The listing builds one solid part. Answer for the finished solid, in the listing's coordinates (mm). A direction names the side the tool comes from. Give positions to 0.01 mm unless a question says otherwise; leave off trailing zeros. Loops run counter-clockwise (first coordinate to the right, second up) from the corner with the lowest first, then second, coordinate; pieces in that order, holes last.
Item 1: Consider line 1 along X through (y, z) = (-26, 5.25); line 2 along Y through (x, z) = (21.5, 3.75); line 3 along Z through (x, y) = (40, -47). Determine where each line is inside the solid, lowest interval first.
Item 2: Section D-D, the plane x = 31.5 is taken. Give the vertices of the cut face in (y, z), and give its area (3 significant figures).
Item 3: Each of these flat-tipped pins is pushed along its axis until it touches: pin 1 Ø5.5 at (x, z) = (35.5, 9) entering from -Y; pin 2 Ø3 at (y, z) = (-17, 20) entering from +X; pin 3 Ø3 at (y, z) = (-47, 20) entering from -X; pin 4 Ø1.1 at (x, y) = (38.5, -44.5) entering from +Z. Where does it stop, or does it pass through?
Item 4: Section C-C, the plane y = 12.4 is taken. Give the vertices of the cut face in (x, z).
Item 5: The mould has two halves that part along Z. Classify faces 1 (the face through (-41.1, -16.6, 0.8)), 2 (the face through (-36.859, -45.014, 3.193)), 3 (the face through (-31.155, 16.362, 19.521)): pulls with the +Z half, pulls with the -Z half, needs draft (parallel to the pull), parting line crosses it, or undercut.
Item 6: A tool of negligible diameter and unlimited length cuts with its end or side. For faces 4 (the face through (-35, 12, 14.6)), 5 (the face through (-36, -9, 11)), 6 (the face through (-38.4, -46, 7.9)), 7 (the face through (30, 17, 19.6)), 8 (the face through (42, -17, 13)), from which of +Z, -Z, +X, -X, +Y, -Y can it reach the whole face along a straight path? Write none if from no direction.
Item 7: Section B-B, the plane x = 13 is taken. Give the vertices of the cut face in (y, z), and give its area (3 significant figures).
Item 8: Section A-A, the plane y = -47 is taken. Give the vertices of the cut face in (x, z), and give its area (3 significant figures).
from build123d import *

# Parameters (mm, degrees)
PAD011_DEPTH    = 23
POCKET004_DEPTH = 5
SKETCH018_R     = 1.25
POCKET005_DEPTH = 84.001
SKETCH019_R     = 1.25
POCKET006_DEPTH = 5
CHAMFER_SIZE    = 1.3
PAD015_DEPTH    = 2
FILLET004_R     = 2.9
FILLET005_R     = 1.9
SKETCH023_W     = 6
SKETCH023_H     = 10
SKETCH023_W_2   = 7
PAD016_DEPTH    = 9
CHAMFER001_SIZE = 8.7
SKETCH024_R     = 1.15
POCKET007_DEPTH = 7


with BuildPart() as part:
    # Sketch015 → Pad011 (new body)
    with BuildSketch(Plane.XY):
        with BuildLine():
            ThreePointArc((-39, 18.5), (-41.12132, 17.62132), (-42, 15.5))
            Line((-42, -51.5), (-42, 15.5))
            Line((-39, -51.5), (-42, -51.5))
            Line((-39, 15.5), (-39, -51.5))
            Line((-39, 15.5), (39, 15.5))
            Line((39, -51.5), (39, 15.5))
            Line((42, -51.5), (39, -51.5))
            Line((42, 15.5), (42, -51.5))
            ThreePointArc((42, 15.5), (41.12132, 17.62132), (39, 18.5))
            Line((-39, 18.5), (39, 18.5))
        make_face()
    extrude(amount=PAD011_DEPTH)

    # Sketch017 (on Face10 of Pad011) → Pocket004 (cut)
    with BuildSketch(Plane(origin=(0, 18.5, 0), x_dir=(-1, 0, 0), z_dir=(0, 1, 0))):
        with BuildLine():
            Line((-25.5, 23), (-25.5, 20.8))
            ThreePointArc((-26.7, 19.6), (-25.851472, 19.951472), (-25.5, 20.8))
            Line((-26.7, 19.6), (-33.8, 19.6))
            ThreePointArc((-35, 20.8), (-34.648528, 19.951472), (-33.8, 19.6))
            Line((-35, 20.8), (-35, 23))
            Line((-35, 23), (-25.5, 23))
        make_face()
    extrude(amount=-POCKET004_DEPTH, mode=Mode.SUBTRACT)

    # Sketch018 (on Face3 of Pocket004) → Pocket005 (cut, through all)
    with BuildSketch(Plane(origin=(-42, 0, 0), x_dir=(0, -1, 0), z_dir=(-1, 0, 0))):
        with Locations((17, 20)):
            Circle(SKETCH018_R)
        with Locations((47, 20)):
            Circle(SKETCH018_R)
    extrude(amount=-POCKET005_DEPTH, mode=Mode.SUBTRACT)

    # Sketch019 (on Face2 of Pocket005) → Pocket006 (cut)
    with BuildSketch(Plane(origin=(0, 18.5, 0), x_dir=(-1, 0, 0), z_dir=(0, 1, 0))):
        with Locations((-13, 20)):
            Circle(SKETCH019_R)
        with Locations((30, 20)):
            Circle(SKETCH019_R)
    extrude(amount=-POCKET006_DEPTH, mode=Mode.SUBTRACT)

    # Chamfer
    chamfer_edges = [part.edges().sort_by_distance(p)[0] for p in [
        (14.25, 18.5, 20),
        (-28.75, 18.5, 20),
        (-42, -45.75, 20),
        (42, -45.75, 20),
        (42, -15.75, 20),
        (-42, -15.75, 20),
    ]]
    chamfer(chamfer_edges, length=CHAMFER_SIZE)

    # Sketch022 (on Face16 of Chamfer) → Pad015 (join)
    with BuildSketch(Plane.XZ.offset(46)):
        with BuildLine():
            Line((38, 17), (39, 17))
            Line((39, 17), (39, 1.99))
            Line((39, 1.99), (34, 1.99))
            ThreePointArc((34, 1.99), (36.828427, 3.161573), (38, 5.99))
            Line((38, 17), (38, 5.99))
        make_face()
        with BuildLine():
            Line((-38, 17), (-39, 17))
            Line((-39, 17), (-39, 1.99))
            Line((-39, 1.99), (-34, 1.99))
            ThreePointArc((-38, 5.99), (-36.828427, 3.161573), (-34, 1.99))
            Line((-38, 17), (-38, 5.99))
        make_face()
    extrude(amount=-PAD015_DEPTH)

    # Fillet004
    fillet004_edges = [part.edges().sort_by_distance(p)[0] for p in [
        (42, -18, 0),
        (41.12132, 17.62132, 0),
        (0, 18.5, 0),
        (-41.12132, 17.62132, 0),
        (-42, -18, 0),
    ]]
    fillet(fillet004_edges, radius=FILLET004_R)

    # Fillet005
    fillet005_edges = [part.edges().sort_by_distance(p)[0] for p in [
        (-42, -51.5, 12.95),
        (42, -51.5, 12.95),
        (41.15061, -51.5, 0.84939),
        (-41.15061, -51.5, 0.84939),
    ]]
    fillet(fillet005_edges, radius=FILLET005_R)

    # Sketch023 (on Face4 of Fillet005) → Pad016 (join)
    with BuildSketch(Plane.YZ.offset(-39)):
        with Locations((-12, 9.6)):
            Rectangle(SKETCH023_W, SKETCH023_H)
        with Locations((12.5, 9.6)):
            Rectangle(SKETCH023_W_2, SKETCH023_H)
    extrude(amount=PAD016_DEPTH)

    # Chamfer001
    chamfer001_edges = [part.edges().sort_by_distance(p)[0] for p in [
        (-30, 12.25, 4.6),
        (-30, -12, 4.6),
    ]]
    chamfer(chamfer001_edges, length=CHAMFER001_SIZE)

    # Sketch024 (on Face26 of Chamfer001) → Pocket007 (cut)
    with BuildSketch(Plane.XY.offset(14.6)):
        with Locations((-32.9, -12)):
            Circle(SKETCH024_R)
        with Locations((-32.9, 12.4)):
            Circle(SKETCH024_R)
    extrude(amount=-POCKET007_DEPTH, mode=Mode.SUBTRACT)


solid = part.part
Worked answers:
1. line 1: x = -42 to -39, 39 to 42
1. line 2: y = 15.5 to 18.5
1. line 3: z = 0.14 to 18.75, 21.25 to 23
2. outline: (15.5, 0) - (15.6, 0) arc R2.9 ccw to (18.5, 2.9) - (18.5, 19.6) - (15.5, 19.6) - close
2. area: 57.0 mm2
3. pin 1: stops at y = -46
3. pin 2: stops at x = 40.95
3. pin 3: stops at x = -40.95
3. pin 4: stops at z = 23
4. outline: (-42, 2.9) arc R2.9 ccw to (-39.1, 0) - (-39, 0) - (-39, 4.6) - (-38.7, 4.6) - (-34.05, 9.25) - (-34.05, 14.6) - (-39, 14.6) - (-39, 23) - (-42, 23) - close; (-31.75, 11.55) - (-30, 13.3) - (-30, 14.6) - (-31.75, 14.6) - close; (39, 0) - (39.1, 0) arc R2.9 ccw to (42, 2.9) - (42, 23) - (39, 23) - close
5. face 1: pulls with the -Z half
5. face 2: pulls with the +Z half
5. face 3: undercut
6. face 4: +Z
6. face 5: +Z, -Z
6. face 6: +Z, -Z, -Y
6. face 7: +Z, +Y, -Y
6. face 8: +Z, -Z, +X, +Y, -Y
7. outline: (15.5, 0) - (15.6, 0) arc R2.9 ccw to (18.5, 2.9) - (18.5, 17.45) - (17.2, 18.75) - (15.5, 18.75) - close; (15.5, 21.25) - (17.2, 21.25) - (18.5, 22.55) - (18.5, 23) - (15.5, 23) - close
7. area: 58.0 mm2
8. outline: (-42, 2.9) arc R2.9 ccw to (-39.1, 0) - (-39, 0) - (-39, 18.75) - (-40.7, 18.75) - (-42, 17.45) - close; (-42, 22.55) - (-40.7, 21.25) - (-39, 21.25) - (-39, 23) - (-42, 23) - close; (39, 0) - (39.1, 0) arc R2.9 ccw to (42, 2.9) - (42, 17.45) - (40.7, 18.75) - (39, 18.75) - close; (39, 21.25) - (40.7, 21.25) - (42, 22.55) - (42, 23) - (39, 23) - close
8. area: 116 mm2
